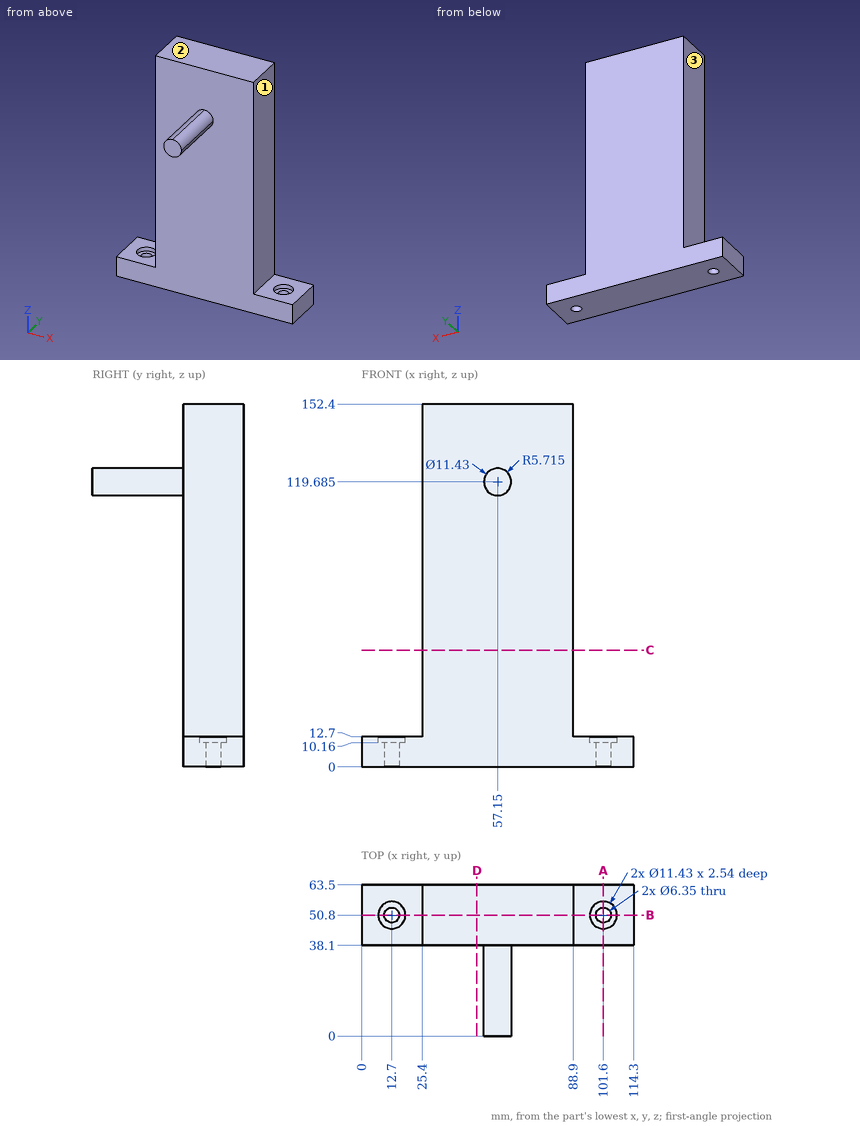
For this review, use the dimensioned drawing (mm, ordinates from the lowest corner) and the shaded views. A direction names the side the tool comes from. Give positions to 0.01 mm unless a question says otherwise; leave off trailing zeros. Write each loop counter-clockwise with the first axis right and the second up, starting at its lowest first coordinate (ties: lowest second). Pieces come first, ordered by that corner, then holes. Notation, with made-up numbers: M 69,77 L 120,77 A15 ccw 120,84 Z; hole C -38,27.25 d8. An arc over 180 degrees is marked long. Answer as a JSON object with one key per item and string values. Group by question number.
Item 1: Tool access review of the marked faces 1, 2 and 3: name each direction out of +Z, -Z, +X, -X, +Y, -Y from which nothing blocks a thin tool from reaching the whole face with its end or side.
Item 2: For pin 1 Ø7.5 at (y, z) = (47.5, 52.5) entering from +X; pin 2 Ø9 at (x, y) = (10.5, 50) entering from +Z; pin 3 Ø7.5 at (x, y) = (12, 49) entering from +Z; pin 4 Ø5.5 at (x, y) = (12.7, 50.8) entering from -Z, all flat-tipped, find the tip position at first contact; note any pin that passes through.
Item 3: Consider section C-C on z = 49. Write out the cut boundary in (x, y).
Item 4: Consider section D-D on x = 48.5. Write out the cut boundary in (y, z), plus the area to 3 significant figures.
Item 5: For probe 1 along Y at (x, z) = (12.7, 4.75) (3 decimals); probe 2 along Y at (x, z) = (101, 12); probe 3 along X at (y, z) = (53, 126.5), list the stretches that pass through material, from the lowest coordinate up. Write a range as [from, to].
Item 6: Consider section A-A on x = 101.6. Write out the cut boundary in (y, z) (3 decimals), plus the area to 3 significant figures.
Item 7: Consider section B-B on y = 50.8. Write out the cut boundary in (x, z) (3 decimals), plus the area to 3 significant figures.
Check result:
{
 "1": {"face 1": "+Z, +X, +Y, -Y", "face 2": "+Z, +X, -X, +Y, -Y", "face 3": "+Z, -X, +Y, -Y"},
 "2": {"pin 1": "stops at x = 88.9", "pin 2": "stops at z = 12.7", "pin 3": "stops at z = 10.16", "pin 4": "passes through"},
 "3": {"outline": "M 25.4,38.1 L 88.9,38.1 L 88.9,63.5 L 25.4,63.5 Z"},
 "4": {"outline": "M 38.1,0 L 63.5,0 L 63.5,152.4 L 38.1,152.4 Z", "area": "3,870 mm^2"},
 "5": {"probe 1": "y = [38.1, 47.625], [53.975, 63.5]", "probe 2": "y = [38.1, 45.12], [56.48, 63.5]", "probe 3": "x = [25.4, 88.9]"},
 "6": {"outline": "M 38.1,0 L 47.625,0 L 47.625,10.16 L 45.085,10.16 L 45.085,12.7 L 38.1,12.7 Z; M 53.975,0 L 63.5,0 L 63.5,12.7 L 56.515,12.7 L 56.515,10.16 L 53.975,10.16 Z", "area": "229 mm^2"},
 "7": {"outline": "M 0,0 L 9.525,0 L 9.525,10.16 L 6.985,10.16 L 6.985,12.7 L 0,12.7 Z; M 15.875,0 L 98.425,0 L 98.425,10.16 L 95.885,10.16 L 95.885,12.7 L 88.9,12.7 L 88.9,152.4 L 25.4,152.4 L 25.4,12.7 L 18.415,12.7 L 18.415,10.16 L 15.875,10.16 Z; M 104.775,0 L 114.3,0 L 114.3,12.7 L 107.315,12.7 L 107.315,10.16 L 104.775,10.16 Z", "area": "10,100 mm^2"}
}
